Verification items for the finished model (mm, model axes). Give positions to 0.01 mm unless a question says otherwise; leave off trailing zeros. Write each loop counter-clockwise with the first axis right and the second up, starting at its lowest first coordinate (ties: lowest second). Pieces come first, ordered by that corner, then holes. Notation, with made-up numbers: (-36.5, -27.75) -> (-20.5, -27.75) arc R25 ccw to (-20.5, -4.75) -> close; hole circle Ø5 at (19, 40). An arc over 180 degrees is marked (long way). Write item = value, one per line.
from build123d import *

# Parameters (mm, degrees)
F0_W        = 101.6
F0_H        = 152.4
F0_W_2      = 20
F0_H_2      = 114.3
F1_DEPTH    = 5
F2_T1_DEPTH = 5


# Not quite as in the source:
# - a fillet or chamfer that OpenCascade refuses, or shapes differently, is made with other operations: its cross-section is extruded or revolved along the edge and cut away or added


with BuildPart() as f1:
    # F0 (on Front) → F1 (new body)
    with BuildSketch(Plane.XZ):
        Rectangle(F0_W, F0_H)
        Rectangle(F0_W_2, F0_H_2, mode=Mode.SUBTRACT)
    extrude(amount=F1_DEPTH)

    # F2: fillet of radius 10.16 on 4 edges, made by hand

    # F2_s2 → F2_t1 (join)
    with BuildSketch(Plane.XZ):
        with BuildLine():
            ThreePointArc((-10, 46.99), (-7.0242048969, 54.1742048969), (0.16, 57.15))
            Line((0.16, 57.15), (-10, 57.15))
            Line((-10, 57.15), (-10, 46.99))
        make_face()
        with BuildLine():
            ThreePointArc((10, 46.99), (7.0242048969, 54.1742048969), (-0.16, 57.15))
            Line((-0.16, 57.15), (10, 57.15))
            Line((10, 57.15), (10, 46.99))
        make_face()
        with BuildLine():
            ThreePointArc((10, -46.99), (7.0242048969, -54.1742048969), (-0.16, -57.15))
            Line((-0.16, -57.15), (10, -57.15))
            Line((10, -57.15), (10, -46.99))
        make_face()
        with BuildLine():
            ThreePointArc((0.16, -57.15), (-7.0242048969, -54.1742048969), (-10, -46.99))
            Line((-10, -46.99), (-10, -57.15))
            Line((-10, -57.15), (0.16, -57.15))
        make_face()
    extrude(amount=F2_T1_DEPTH)


solid = f1.part
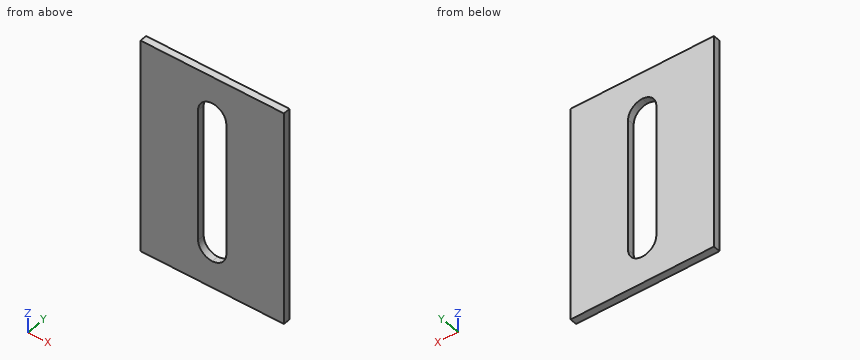
Item 1: Sectioned sample at B-B on y = -3.8. Record the cut outline in (x, z).
Response values:
outline = (-50.8, -76.2) -> (50.8, -76.2) -> (50.8, 76.2) -> (-50.8, 76.2) -> close; hole (-10, -46.99) arc R10.16 ccw to (0, -57.15) arc R10.16 ccw to (10, -46.99) -> (10, 46.99) arc R10.16 ccw to (0, 57.15) arc R10.16 ccw to (-10, 46.99) -> close
Item 2: Material ranges on line 1 (X direction, y = -0.85, z = -17); line 2 (Z direction, x = 6, y = -2.5); line 3 (Z direction, x = -2.5, y = -4.1), recorded low to high.
Response values:
line_1 = -50.8 to -10, 10 to 50.8
line_2 = -76.2 to -55.07, 55.07 to 76.2
line_3 = -76.2 to -56.8, 56.8 to 76.2
Item 3: Sectioned sample at C-C on x = 5.5. Record the cut outline in (y, z).
Response values:
outline = (-5, -76.2) -> (0, -76.2) -> (0, -55.43) -> (-5, -55.43) -> close; (-5, 55.43) -> (0, 55.43) -> (0, 76.2) -> (-5, 76.2) -> close
Item 4: Sectioned sample at A-A on z = 45.5. Record the cut outline in (x, y), then the cut area to 3 significant figures.
Response values:
outline = (-50.8, -5) -> (-10, -5) -> (-10, 0) -> (-50.8, 0) -> close; (10, -5) -> (50.8, -5) -> (50.8, 0) -> (10, 0) -> close
area = 408 mm^2
Item 5: Go/stop test with a flat-tipped pin: P1, Ø6, axis at x = 17.5, z = -45.5, coming from the +Y side. Record where the tip stops, or that it passes through.
Response values:
P1 = 0
